Can you work these out from the drawing? Everything is in mm from the part's minimum corner. A direction names the side the tool comes from. Coordinates: 2 decimals unless noted, no trailing zeros. Loops run counter-clockwise (first coordinate to the right, second up) from the corner with the lowest first, then second, coordinate; pieces in that order, holes last.
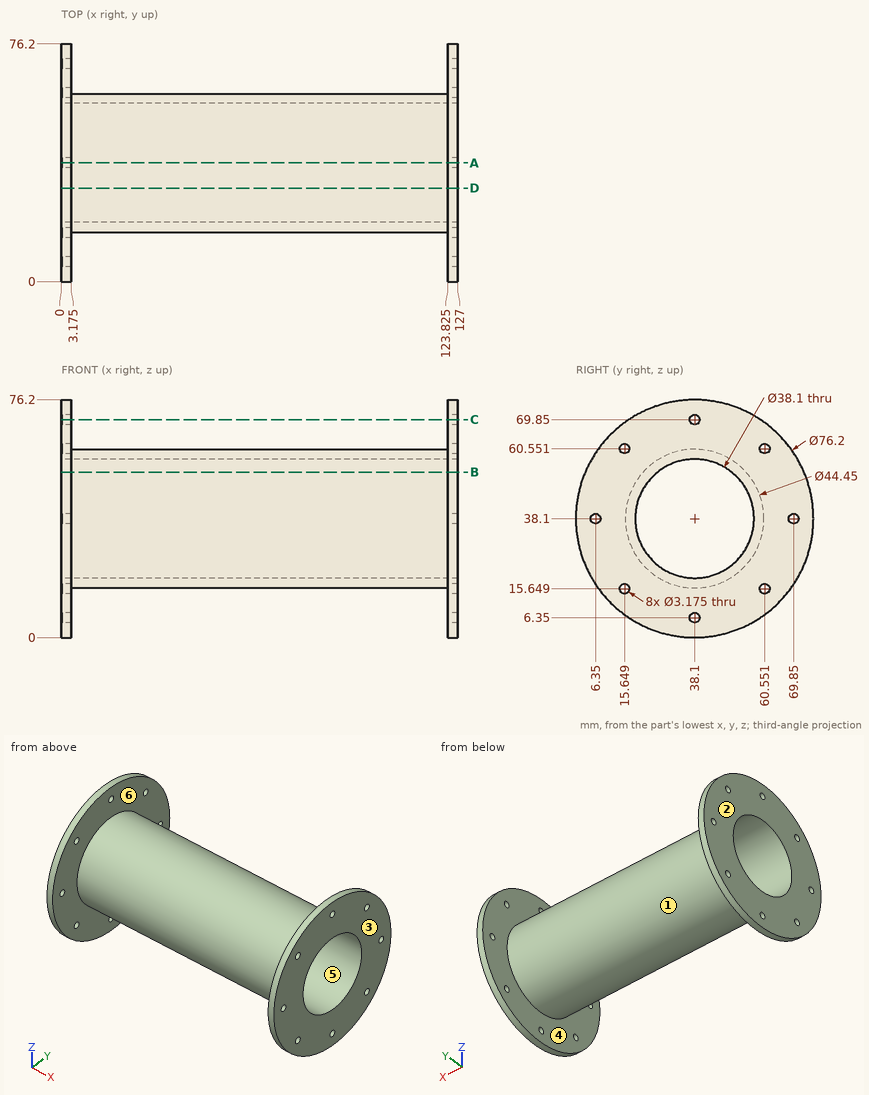
(1) Imagine slicing it at D-D, the plane y = 30. Write out the boundary of the cut face in (x, z) (1 decimal), and give its area (3 significant figures).
Answers:
outline: (0, 0.9) - (3.2, 0.9) - (3.2, 17.4) - (123.8, 17.4) - (123.8, 0.9) - (127, 0.9) - (127, 20.9) - (0, 20.9) - close; (0, 55.3) - (127, 55.3) - (127, 75.3) - (123.8, 75.3) - (123.8, 58.8) - (3.2, 58.8) - (3.2, 75.3) - (0, 75.3) - close
area: 1,090 mm2
(2) Imagine slicing it at A-A, the plane y = 38.1. State how many separate pieces and enclosed holes the cut face has.
Answers:
separate pieces: 6
enclosed holes: 0
(3) For pin 1 (3 mm diameter, centred on y = 15.65, z = 15.65, fed in from +X); pin 2 (4 mm diameter, centred on x = 37.5, z = 29, fed in from +Y); pin 3 (4 mm diameter, centred on x = 67, z = 19, fed in from +Y) (1 decimal); pin 4 (3 mm diameter, centred on x = 49.5, z = 55.5, fed in from +Y), each with a flat end and sliding along its axis, tell me the tip position at first contact or that it passes through.
Answers:
pin 1: passes through
pin 2: stops at y = 59.16
pin 3: stops at y = 52.3
pin 4: stops at y = 53.63
(4) We'd pull the mould along X, two halves only. Please class the marked faces 3, 4, 5 and 6: +X half, -X half, draft (parallel to the pull), parting line (faces both ways), or undercut.
Answers:
face 3: +X half
face 4: undercut
face 5: draft
face 6: undercut
(5) Which directions (+Z, -Z, +X, -X, +Y, -Y) give clear straight access to the entire face, cutting with the end or side of a thin tool? Please do the marked faces 1 and 2.
Answers:
face 1: none
face 2: +Z, -Z, -X, +Y, -Y
(6) Imagine slicing it at C-C, the plane z = 69.85. Write out the boundary of the cut face in (x, y) (1 decimal).
Answers:
outline: (0, 17) - (3.2, 17) - (3.2, 36.5) - (0, 36.5) - close; (0, 39.7) - (3.2, 39.7) - (3.2, 59.2) - (0, 59.2) - close; (123.8, 17) - (127, 17) - (127, 36.5) - (123.8, 36.5) - close; (123.8, 39.7) - (127, 39.7) - (127, 59.2) - (123.8, 59.2) - close
(7) I need wall thicknesses on probe 1 along Z at (x, y) = (1.1, 38.1); probe 2 along X at (y, z) = (42, 67.5) (1 decimal); probe 3 along Z at (x, y) = (43.5, 24.5). Which ranges of each line are inside material? Lowest first, please.
Answers:
probe 1: z = 0 to 4.76, 7.94 to 19.05, 57.15 to 68.26, 71.44 to 76.2
probe 2: x = 0 to 3.2, 123.8 to 127
probe 3: z = 20.52 to 24.76, 51.44 to 55.68
(8) Imagine slicing it at B-B, the plane z = 53. Write out the boundary of the cut face in (x, y) (1 decimal), and give its area (3 significant figures).
Answers:
outline: (0, 3) - (3.2, 3) - (3.2, 21.6) - (123.8, 21.6) - (123.8, 3) - (127, 3) - (127, 26.2) - (0, 26.2) - close; (0, 50) - (127, 50) - (127, 73.2) - (123.8, 73.2) - (123.8, 54.6) - (3.2, 54.6) - (3.2, 73.2) - (0, 73.2) - close
area: 1,410 mm2
